Verification items for the finished model (mm, model axes). Face numbers are marked on the shaded views. A direction names the side the tool comes from. Round coordinates to 2 decimals unless told otherwise and drop trailing zeros. Write each loop counter-clockwise with the first axis right and the second up, starting at its lowest first coordinate (ties: lowest second). Pieces come first, ordered by that corner, then holes. Notation, with made-up numbers: M 63,5.25 L 69,5.25 A25 ccw 69,24.25 Z; hole C -23,59 d1. An arc over 180 degrees is marked long. Answer in a Markdown table with one row per item. Add a question column.
1. Sectioned sample at C-C on z = 0.2. Record the cut outline in (x, y), plus the area to 3 significant figures.
2. Sectioned sample at A-A on x = 0. Record the cut outline in (y, z), plus the area to 3 significant figures.
3. Draft check along Y on the marked faces 3 and 4. Enter one of: pulls with the +Y half, pulls with the -Y half, needs draft (parallel to the pull), parting line crosses it, or undercut.
4. Set-up check for the marked faces 1 and 2: record each of +Z, -Z, +X, -X, +Y, -Y from which the full face is reachable in a straight line by a thin tool's end or side.
5. Material ranges on probe 1 along Y at (x, z) = (0, -0.1); probe 2 along Z at (x, y) = (3, 0.5); probe 3 along Y at (x, z) = (-1.75, -0.85), recorded low to high.
6. Go/stop test with flat-tipped pins: pin 1 Ø2 at (x, y) = (-3.5, 3) entering from +Z; pin 2 Ø1.5 at (y, z) = (-1, -2) entering from -X; pin 3 Ø1 at (y, z) = (-3.5, -1.5) entering from +X. Record where each tip stops, or that it passes through.
7. Sectioned sample at D-D on z = -1.85. Record the cut outline in (x, y).
```python
from build123d import *

# Parameters (mm, degrees)
F2_R     = 2
F3_DEPTH = 5


with BuildPart() as f1:
    # F0 (on Front) → F1 (revolve)
    with BuildSketch(Plane.XZ):
        with BuildLine():
            Line((0, 2.5), (0, 0))
            Line((0, 0), (0, -2.5))
            Line((0, -2.5), (3, -2.5))
            ThreePointArc((3, -2.5), (4.06066, -2.06066), (4.5, -1))
            Line((4.5, -1), (4.5, -0.75))
            Line((4.5, -0.75), (3, -0.75))
            Line((3, -0.75), (3, 0.75))
            Line((3, 0.75), (4.5, 0.75))
            Line((4.5, 0.75), (4.5, 1))
            ThreePointArc((4.5, 1), (4.06066, 2.06066), (3, 2.5))
            Line((3, 2.5), (0, 2.5))
        make_face()
    revolve(axis=Axis((0, 0, 1.25), (0, 0, 1)))

    # F2 (on face) → F3 (cut, through all)
    with BuildSketch(Plane.XY.offset(2.5)):
        Circle(F2_R)
    extrude(amount=-F3_DEPTH, mode=Mode.SUBTRACT)


solid = f1.part
```
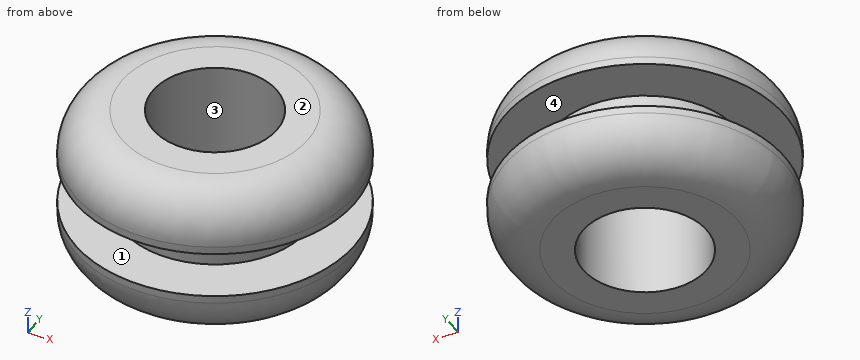
Geometry check:
| question | item | result |
|---|---|---|
| 1 | outline | C 0,0 d6; hole C 0,0 d4 |
| 1 | area | 15.7 mm2 |
| 2 | outline | M -4.5,-1 A1.5 ccw -3,-2.5 L -2,-2.5 L -2,2.5 L -3,2.5 A1.5 ccw -4.5,1 L -4.5,0.75 L -3,0.75 L -3,-0.75 L -4.5,-0.75 Z; M 2,-2.5 L 3,-2.5 A1.5 ccw 4.5,-1 L 4.5,-0.75 L 3,-0.75 L 3,0.75 L 4.5,0.75 L 4.5,1 A1.5 ccw 3,2.5 L 2,2.5 Z |
| 2 | area | 18.6 mm2 |
| 3 | face 3 | undercut |
| 3 | face 4 | needs draft |
| 4 | face 1 | none |
| 4 | face 2 | +Z, +X, -X, +Y, -Y |
| 5 | probe 1 | y = -3 to -2, 2 to 3 |
| 5 | probe 2 | z = -2.5 to -0.75, 0.75 to 2.5 |
| 5 | probe 3 | y = -4.15 to -0.97, 0.97 to 4.15 |
| 6 | pin 1 | stops at z = 2.37 |
| 6 | pin 2 | stops at x = -4.41 |
| 6 | pin 3 | stops at x = 3.28 |
| 7 | outline | C 0,0 d8.47; hole C 0,0 d4 |
